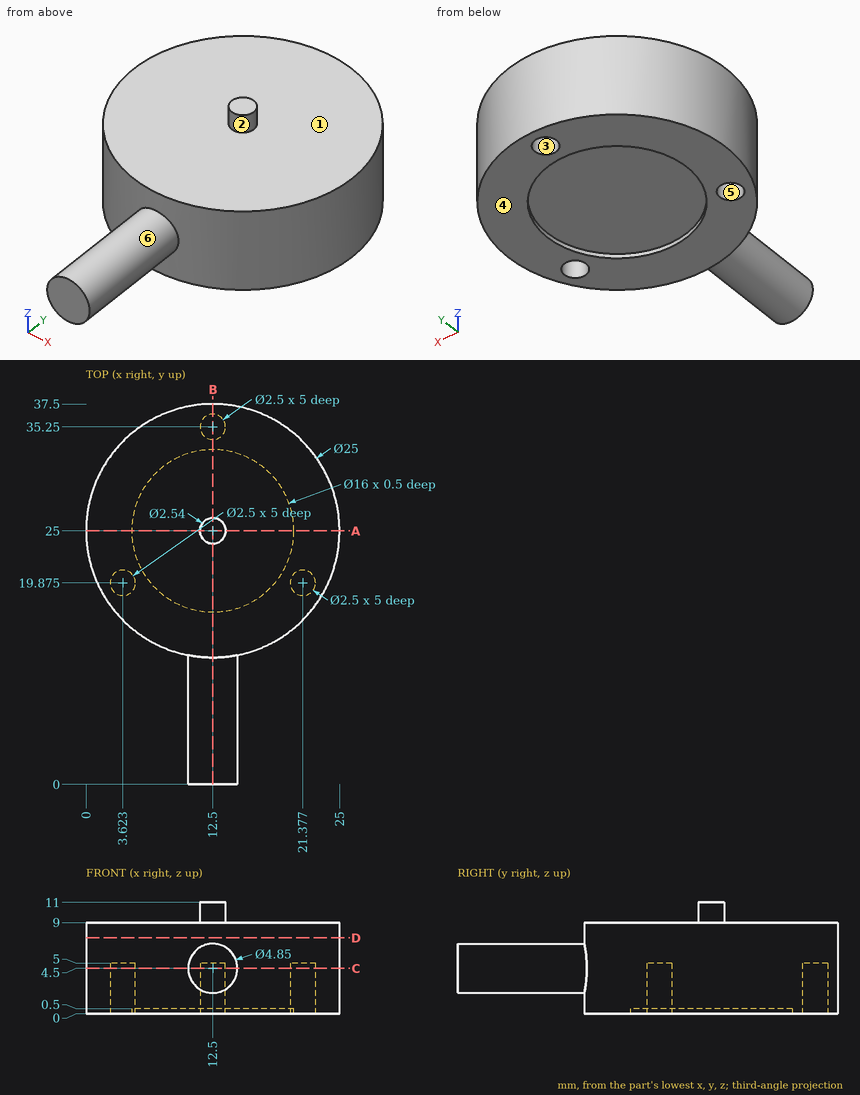
Verification items for this drawing (mm, ordinates from the low corner). A direction names the side the tool comes from. Coordinates: 2 decimals unless noted, no trailing zeros. Order: outer loops, then holes, each group sorted by start corner. A loop starts at its lowest first (then second) coordinate and runs counter-clockwise, first axis right, second up.
Q1. Sectioned sample at D-D on z = 7.5. Record the cut outline in (x, y), and give its area (3 significant figures).
Reply:
outline: circle Ø25 at (12.5, 25)
area: 491 mm2
Q2. Depth check by flat-ended pin: pin 1 Ø6 at (y, z) = (8.5, 4.5) entering from -X (3 decimals); pin 2 Ø12.5 at (x, y) = (15, 23) entering from +Z; pin 3 Ø4 at (x, z) = (8, 9) entering from -Y; pin 4 Ø1 at (x, y) = (9, 25) entering from +Z. Enter the tip coordinate at first touch or a pass-through.
Reply:
pin 1: stops at x = 10.075
pin 2: stops at z = 11
pin 3: stops at y = 12.75
pin 4: stops at z = 9
Q3. Sectioned sample at B-B on x = 12.5. Record the cut outline in (y, z) (3 decimals), and give its area (3 significant figures).
Reply:
outline: (0, 2.075) - (12.5, 2.075) - (12.5, 0) - (17, 0) - (17, 0.5) - (33, 0.5) - (33, 0) - (34, 0) - (34, 5) - (36.5, 5) - (36.5, 0) - (37.5, 0) - (37.5, 9) - (26.27, 9) - (26.27, 11) - (23.73, 11) - (23.73, 9) - (12.5, 9) - (12.5, 6.925) - (0, 6.925) - close
area: 270 mm2
Q4. Sectioned sample at C-C on z = 4.5. Give the number of separate pieces and of enclosed holes in the cut face, and give its area (3 significant figures).
Reply:
separate pieces: 1
enclosed holes: 3
area: 537 mm2
Q5. Draft check along Y on the marked faces 1, 2 and 3. Enter one of: released by +Y, released by -Y, zero draft, split by the parting line, or undercut.
Reply:
face 1: zero draft
face 2: split by the parting line
face 3: undercut
Q6. Thickness scan on probe 1 along Y at (x, z) = (12.5, 0.2); probe 2 along Y at (x, z) = (12.5, 2.75); probe 3 along Z at (x, y) = (19.25, 30). Record the ranges inside material, lowest first.
Reply:
probe 1: y = 12.5 to 17, 33 to 34, 36.5 to 37.5
probe 2: y = 0 to 34, 36.5 to 37.5
probe 3: z = 0 to 9
Q7. Tool access check on the marked faces 4, 5 and 6. Record the directions out of +Z, -Z, +X, -X, +Y, -Y that give a thin tool (end or side, any length) a straight path to the whole face; none if there is none.
Reply:
face 4: -Z, +X, -X, +Y, -Y
face 5: -Z
face 6: -Y
Q8. Sectioned sample at A-A on y = 25. Record the cut outline in (x, z), and give its area (3 significant figures).
Reply:
outline: (0, 0) - (4.5, 0) - (4.5, 0.5) - (20.5, 0.5) - (20.5, 0) - (25, 0) - (25, 9) - (13.77, 9) - (13.77, 11) - (11.23, 11) - (11.23, 9) - (0, 9) - close
area: 222 mm2
